Here's how the part is built. I have some questions about the finished solid (model axes, mm). Face numbers are marked on the shaded views. A direction names the side the tool comes from. Give positions to 0.01 mm unless a question says otherwise; leave off trailing zeros. Loops run counter-clockwise (first coordinate to the right, second up) from the corner with the lowest first, then second, coordinate; pieces in that order, holes last. Notation, with made-up numbers: (-28.75, 23.25) -> (-6.75, 23.25) arc R21 ccw to (-6.75, 51.25) -> close; hole circle Ø11 at (-18.5, -6.75). An arc over 180 degrees is marked (long way). Answer in a Markdown table with one row per item. Add a question column.
Item 1: If we section it at C-C (z = 13.5): Write out the boundary of the cut face in (x, y), then the cut area to 3 significant figures.
Item 2: For P1, Ø1, axis at x = -3, y = 5, coming from the -Z side; P2, Ø3, axis at x = 0, z = 0, coming from the +Y side; P3, Ø4, axis at x = 0.5, z = 3.5, coming from the +Y side (3 decimals), each with a flat end and sliding along its axis, tell me the tip position at first contact or that it passes through.
Item 3: Which directions (+Z, -Z, +X, -X, +Y, -Y) give clear straight access to the entire face, cutting with the end or side of a thin tool? Please do the marked faces 1 and 2.
Item 4: If I drill on line 1 (Y direction, x = 0, z = 15); line 2 (X direction, y = 1.75, z = 0); line 3 (Y direction, x = 0.5, z = 5.75) (3 decimals), over which ranges is the centre line in solid material (lowest first)?
Item 5: We'd pull the mould along Y, two halves only. Please class the marked faces 3, 4 and 5: released by +Y, released by -Y, zero draft, split by the parting line, or undercut.
Item 6: If we section it at D-D (y = 7.75): Write out the boundary of the cut face in (x, z) (3 decimals), then the cut area to 3 significant figures.
Item 7: If we section it at A-A (x = 0): Write out the boundary of the cut face in (y, z) (3 decimals).
Item 8: If we section it at B-B (y = 1.5): Write out the boundary of the cut face in (x, z) (3 decimals), then the cut area to 3 significant figures.
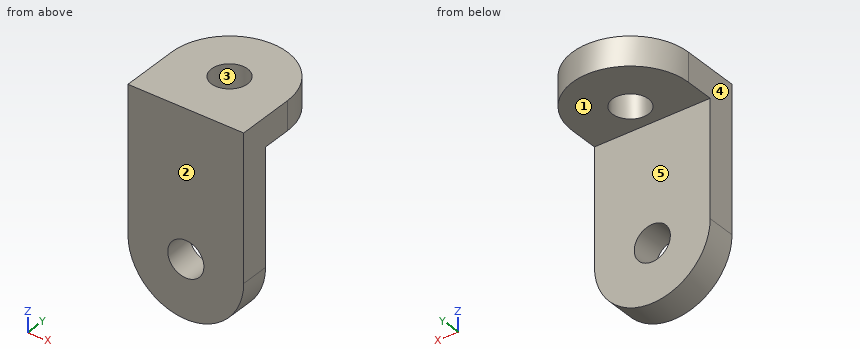
Autodesk Inventor part; units mm, degrees
ref_plane "YZ Plane" through (0, 0, 0) normal (1, 0, 0) x (0, 1, 0)
ref_plane "XZ Plane" through (0, 0, 0) normal (0, 1, 0) x (-1, 0, 0)
ref_plane "XY Plane" through (0, 0, 0) normal (0, 0, 1) x (1, 0, 0)
sketch "Sketch1" plane through (0, 0, 0) normal (0, 1, 0) x (-1, 0, 0)
  circle A0 centre (0, 0) radius 6.35
  line L0 (6.35, 0) -> (6.35, 12.7)
  line L1 (6.35, 12.7) -> (-6.35, 12.7)
  line L2 (-6.35, 12.7) -> (-6.35, 0)
  dimension "d0" = 12.7
  dimension "d1" = 12.7
extrude "Extrusion1" add sketch "Sketch1" along normal blind 3.175
sketch "Sketch2" plane through (-6.35, 0, 12.7) normal (0, 0, 1) x (1, 0, 0)
  circle A0 centre (6.35, 6.35) radius 6.35
  line L0 (0, 6.35) -> (0, 0)
  line L1 (0, 0) -> (12.7, 0)
  line L2 (0, 0) -> (12.7, 0)
  line L3 (12.7, 0) -> (12.7, 6.35)
  point P0 (6.35, 0)
  dimension "d4" = 12.7
  dimension "d5" = 6.35
extrude "Extrusion2" add sketch "Sketch2" along normal blind 3.175
hole "Hole1" at (0, 0, 0) direction (0, 1, 0) diameter 3.9624 depth 13.6144
hole "Hole2" at (0, 6.35, 12.7) direction (0, 0, 1) diameter 3.9624 end through all
properties part number "Rotational Linkage"
Recorded:
| question | item | result |
|---|---|---|
| 1 | outline | (-6.35, 0) -> (6.35, 0) -> (6.35, 6.35) arc R6.35 ccw to (-6.35, 6.35) -> close; hole circle Ø3.96 at (0, 6.35) |
| 1 | area | 132 mm^2 |
| 2 | P1 | stops at z = 12.7 |
| 2 | P2 | passes through |
| 2 | P3 | stops at y = 3.175 |
| 3 | face 1 | -Z, +X, -X, +Y |
| 3 | face 2 | +Z, -Z, +X, -X, -Y |
| 4 | line 1 | y = 0 to 4.37, 8.33 to 12.7 |
| 4 | line 2 | x = -6.35 to -1.98, 1.98 to 6.35 |
| 4 | line 3 | y = 0 to 3.175 |
| 5 | face 3 | undercut |
| 5 | face 4 | zero draft |
| 5 | face 5 | released by +Y |
| 6 | outline | (-6.194, 12.7) -> (-1.402, 12.7) -> (-1.402, 15.875) -> (-6.194, 15.875) -> close; (1.402, 12.7) -> (6.194, 12.7) -> (6.194, 15.875) -> (1.402, 15.875) -> close |
| 6 | area | 30.4 mm^2 |
| 7 | outline | (0, -6.35) -> (3.175, -6.35) -> (3.175, -1.981) -> (0, -1.981) -> close; (0, 1.981) -> (3.175, 1.981) -> (3.175, 12.7) -> (4.369, 12.7) -> (4.369, 15.875) -> (0, 15.875) -> close; (8.331, 12.7) -> (12.7, 12.7) -> (12.7, 15.875) -> (8.331, 15.875) -> close |
| 8 | outline | (-6.35, 0) arc R6.35 ccw to (6.35, 0) -> (6.35, 15.875) -> (-6.35, 15.875) -> close; hole circle Ø3.962 at (0, 0) |
| 8 | area | 253 mm^2 |
